Could you check a few things on this model? Use its own coordinates, in mm. A direction names the side the tool comes from. Give positions to 0.01 mm unless a question says otherwise; leave off trailing zeros. Loops run counter-clockwise (first coordinate to the right, second up) from the corner with the lowest first, then second, coordinate; pieces in that order, holes last.
1. For faces 4 (the conical face through (-17.686, 1.125, -29.712)), 5 (the cylindrical face through (19.122, 1.479, 33.174)), which set-ups out of +Z, -Z, +X, -X, +Y, -Y let a thin tool reach every point of the face, with its end or its side?
2. Imagine slicing it at D-D (z = -18). List the corners of the cut face in (x, y) for me.
3. I need wall thicknesses on line 1 along X through (y, z) = (1.45, -24.5); line 2 along X through (y, z) = (1.05, -18); line 3 along Z through (x, y) = (-15, 1.05). Which ranges of each line are inside material? Lowest first, please.
4. For P1, Ø2.5, axis at x = -32.5, z = 0, coming from the -Y side; P2, Ø6.5, axis at x = -16.25, z = 28.15, coming from the +Y side; P3, Ø4, axis at x = 42.44, z = 24.5, coming from the -Y side, each with a flat end and sliding along its axis, tell me the tip position at first contact or that it passes through.
5. Imagine slicing it at A-A (z = 0). List the corners of the cut face in (x, y) for me.
6. Thinking about a two-plate mould opening in X: for faces 1 (the flat face through (14, 1.52, -39.17)), 2 (the flat face through (3.12, 1.52, -36.86)), 3 (the flat face through (-22, 3, 22)), which applies, +X half, -X half, draft (parallel to the pull), parting line (faces both ways), or undercut?
7. Imagine slicing it at C-C (z = 49). List the corners of the cut face in (x, y) for me (3 decimals).
8. Imagine slicing it at B-B (x = -16.25). List the corners of the cut face in (y, z) for me.
```python
from build123d import *

# Parameters (mm, degrees)
SKETCH_1_R               = 52
SKETCH_1_R_2             = 1.525
SKETCH_1_R_3             = 2
SKETCH_1_R_4             = 27.5
EXTRUDE_1_DEPTH          = 3
HOLE_WIZARD_1_AT_2_COUNT = 2
HOLE_WIZARD_1_AT_2_PITCH = 32.5
HOLE_WIZARD_1_AT_3_COUNT = 2
HOLE_WIZARD_1_AT_3_PITCH = 56.291651246
HOLE_WIZARD_1_AT_4_COUNT = 2
HOLE_WIZARD_1_AT_4_PITCH = 65
HOLE_WIZARD_1_AT_5_COUNT = 2
HOLE_WIZARD_1_AT_5_PITCH = 56.291651246
HOLE_WIZARD_1_AT_6_COUNT = 2
HOLE_WIZARD_1_AT_6_PITCH = 32.5
CUT_EXTRUDE_1_DEPTH      = 10
FILLET_1_R               = 5
FILLET_2_R               = 1


with BuildPart() as part:
    # 草图1 → 凸台-拉伸1 (new body)
    with BuildSketch(Plane(origin=(0, 0, 0), x_dir=(1, 0, 0), z_dir=(0, 1, 0))):
        with Locations(Location((0, 0, 0), (0, 0, 270))):
            Circle(SKETCH_1_R)
        with Locations(Location((0, 49, 0), (0, 0, 270))):
            Circle(SKETCH_1_R_2, mode=Mode.SUBTRACT)
        with Locations(Location((-16.25, 28.145825623, 0), (0, 0, 270))):
            Circle(SKETCH_1_R_3, mode=Mode.SUBTRACT)
        with Locations(Location((42.435244785, 24.5, 0), (0, 0, 270))):
            Circle(SKETCH_1_R_2, mode=Mode.SUBTRACT)
        with Locations(Location((16.25, 28.145825623, 0), (0, 0, 270))):
            Circle(SKETCH_1_R_3, mode=Mode.SUBTRACT)
        with Locations(Location((42.435244785, -24.5, 0), (0, 0, 270))):
            Circle(SKETCH_1_R_2, mode=Mode.SUBTRACT)
        with Locations(Location((32.5, 0, 0), (0, 0, 270))):
            Circle(SKETCH_1_R_3, mode=Mode.SUBTRACT)
        with Locations(Location((0, -49, 0), (0, 0, 270))):
            Circle(SKETCH_1_R_2, mode=Mode.SUBTRACT)
        with Locations(Location((16.25, -28.145825623, 0), (0, 0, 270))):
            Circle(SKETCH_1_R_3, mode=Mode.SUBTRACT)
        with Locations(Location((-42.435244785, -24.5, 0), (0, 0, 270))):
            Circle(SKETCH_1_R_2, mode=Mode.SUBTRACT)
        with Locations(Location((-16.25, -28.145825623, 0), (0, 0, 270))):
            Circle(SKETCH_1_R_3, mode=Mode.SUBTRACT)
        with Locations(Location((-42.435244785, 24.5, 0), (0, 0, 270))):
            Circle(SKETCH_1_R_2, mode=Mode.SUBTRACT)
        with Locations(Location((-32.5, 0, 0), (0, 0, 270))):
            Circle(SKETCH_1_R_3, mode=Mode.SUBTRACT)
        with Locations(Location((0, 0, 0), (0, 0, 270))):
            Circle(SKETCH_1_R_4, mode=Mode.SUBTRACT)
    extrude(amount=EXTRUDE_1_DEPTH)

    # 草图3 → 孔1 (revolve, cut)
    with BuildSketch(Plane(origin=(-16.25, 3, -28.145825623), x_dir=(0, 0, 1), z_dir=(1, 0, 0))):
        Polygon((0, 0), (0, 3), (2, 3), (2, 2), (4, 0), align=None)
    hole_wizard_1 = revolve(axis=Axis((-16.25, 9.445314094, -28.145825623), (0, -1, 0)), mode=Mode.SUBTRACT)

    # 孔1 at 2: 孔1 ×2
    with Locations(*[(i * HOLE_WIZARD_1_AT_2_PITCH, 0, 0) for i in range(1, HOLE_WIZARD_1_AT_2_COUNT)]):
        add(hole_wizard_1, mode=Mode.SUBTRACT)

    # 孔1 at 3: 孔1 ×2
    with Locations(*[Vector(0.8660254037844387, 0, 0.5) * (i * HOLE_WIZARD_1_AT_3_PITCH) for i in range(1, HOLE_WIZARD_1_AT_3_COUNT)]):
        add(hole_wizard_1, mode=Mode.SUBTRACT)

    # 孔1 at 4: 孔1 ×2
    with Locations(*[Vector(0.5000000000000001, 0, 0.8660254037844386) * (i * HOLE_WIZARD_1_AT_4_PITCH) for i in range(1, HOLE_WIZARD_1_AT_4_COUNT)]):
        add(hole_wizard_1, mode=Mode.SUBTRACT)

    # 孔1 at 5: 孔1 ×2
    with Locations(*[(0, 0, i * HOLE_WIZARD_1_AT_5_PITCH) for i in range(1, HOLE_WIZARD_1_AT_5_COUNT)]):
        add(hole_wizard_1, mode=Mode.SUBTRACT)

    # 孔1 at 6: 孔1 ×2
    with Locations(*[Vector(-0.5000000000000003, 0, 0.8660254037844386) * (i * HOLE_WIZARD_1_AT_6_PITCH) for i in range(1, HOLE_WIZARD_1_AT_6_COUNT)]):
        add(hole_wizard_1, mode=Mode.SUBTRACT)

    # 草图5 → 切除-拉伸1 (cut)
    with BuildSketch(Plane(origin=(0, 3, 0), x_dir=(1, 0, 0), z_dir=(0, 1, 0))):
        with BuildLine():
            Line((-8.501262172, 46.22476113), (-18.947738206, 32.818445262))
            Line((-18.947738206, 32.818445262), (-35.781186336, 30.47468957))
            ThreePointArc((-35.781186336, 30.47468957), (-23.5, 40.703193978), (-8.501262172, 46.22476113))
        make_face()
        with BuildLine():
            Line((0, 40.865281716), (7.136483547, 31.706791111))
            ThreePointArc((7.136483547, 31.706791111), (0, 32.5), (-7.136483547, 31.706791111))
            Line((-7.136483547, 31.706791111), (0, 40.865281716))
        make_face()
        with BuildLine():
            Line((18.947738206, 32.818445262), (8.501262172, 46.22476113))
            ThreePointArc((8.501262172, 46.22476113), (23.5, 40.703193978), (35.781186336, 30.47468957))
            Line((35.781186336, 30.47468957), (18.947738206, 32.818445262))
        make_face()
        with BuildLine():
            Line((35.390372099, 20.432640858), (23.890644801, 22.033771601))
            ThreePointArc((23.890644801, 22.033771601), (28.145825623, 16.25), (31.027128348, 9.67301951))
            Line((31.027128348, 9.67301951), (35.390372099, 20.432640858))
        make_face()
        with BuildLine():
            Line((37.895476413, 0), (44.282448508, 15.75007156))
            ThreePointArc((44.282448508, 15.75007156), (47, 0), (44.282448508, -15.75007156))
            Line((44.282448508, -15.75007156), (37.895476413, 0))
        make_face()
        with BuildLine():
            Line((35.390372099, -20.432640858), (31.027128348, -9.67301951))
            ThreePointArc((31.027128348, -9.67301951), (28.145825623, -16.25), (23.890644801, -22.033771601))
            Line((23.890644801, -22.033771601), (35.390372099, -20.432640858))
        make_face()
        with BuildLine():
            Line((18.947738206, -32.818445262), (35.781186336, -30.47468957))
            ThreePointArc((35.781186336, -30.47468957), (23.5, -40.703193978), (8.501262172, -46.22476113))
            Line((8.501262172, -46.22476113), (18.947738206, -32.818445262))
        make_face()
        with BuildLine():
            Line((0, -40.865281716), (7.136483547, -31.706791111))
            ThreePointArc((7.136483547, -31.706791111), (0, -32.5), (-7.136483547, -31.706791111))
            Line((-7.136483547, -31.706791111), (0, -40.865281716))
        make_face()
        with BuildLine():
            Line((-18.947738206, -32.818445262), (-8.501262172, -46.22476113))
            ThreePointArc((-8.501262172, -46.22476113), (-23.5, -40.703193978), (-35.781186336, -30.47468957))
            Line((-35.781186336, -30.47468957), (-18.947738206, -32.818445262))
        make_face()
        with BuildLine():
            Line((-35.390372099, -20.432640858), (-23.890644801, -22.033771601))
            ThreePointArc((-23.890644801, -22.033771601), (-28.145825623, -16.25), (-31.027128348, -9.67301951))
            Line((-31.027128348, -9.67301951), (-35.390372099, -20.432640858))
        make_face()
        with BuildLine():
            Line((-37.895476413, 0), (-44.282448508, -15.75007156))
            ThreePointArc((-44.282448508, -15.75007156), (-47, 0), (-44.282448508, 15.75007156))
            Line((-44.282448508, 15.75007156), (-37.895476413, 0))
        make_face()
        with BuildLine():
            Line((-35.390372099, 20.432640858), (-31.027128348, 9.67301951))
            ThreePointArc((-31.027128348, 9.67301951), (-28.145825623, 16.25), (-23.890644801, 22.033771601))
            Line((-23.890644801, 22.033771601), (-35.390372099, 20.432640858))
        make_face()
    extrude(amount=-CUT_EXTRUDE_1_DEPTH, mode=Mode.SUBTRACT)

    # 圆角1
    fillet_1_edges = [part.edges().sort_by_distance(p)[0] for p in [
        (-18.947738206, 1.5, 32.818445262),
        (18.947738206, 1.5, 32.818445262),
        (37.895476413, 1.5, 0),
        (18.947738206, 1.5, -32.818445262),
        (-37.895476413, 1.5, 0),
        (-18.947738206, 1.5, -32.818445262),
    ]]
    fillet(fillet_1_edges, radius=FILLET_1_R)

    # 圆角2
    fillet_2_edges = [part.edges().sort_by_distance(p)[0] for p in [
        (-8.501262172, 1.5, 46.22476113),
        (-35.781186336, 1.5, 30.47468957),
        (0, 1.5, 40.865281716),
        (-7.136483547, 1.5, 31.706791111),
        (7.136483547, 1.5, 31.706791111),
        (35.781186336, 1.5, 30.47468957),
        (8.501262172, 1.5, 46.22476113),
        (35.390372099, 1.5, 20.432640858),
        (23.890644801, 1.5, 22.033771601),
        (31.027128348, 1.5, 9.67301951),
        (44.282448508, 1.5, -15.75007156),
        (44.282448508, 1.5, 15.75007156),
        (35.390372099, 1.5, -20.432640858),
        (31.027128348, 1.5, -9.67301951),
        (23.890644801, 1.5, -22.033771601),
        (8.501262172, 1.5, -46.22476113),
        (35.781186336, 1.5, -30.47468957),
        (-7.136483547, 1.5, -31.706791111),
        (0, 1.5, -40.865281716),
        (7.136483547, 1.5, -31.706791111),
        (-35.390372099, 1.5, -20.432640858),
        (-23.890644801, 1.5, -22.033771601),
        (-31.027128348, 1.5, -9.67301951),
        (-44.282448508, 1.5, 15.75007156),
        (-44.282448508, 1.5, -15.75007156),
        (-35.390372099, 1.5, 20.432640858),
        (-31.027128348, 1.5, 9.67301951),
        (-23.890644801, 1.5, 22.033771601),
        (-35.781186336, 1.5, -30.47468957),
        (-8.501262172, 1.5, -46.22476113),
    ]]
    fillet(fillet_2_edges, radius=FILLET_2_R)


solid = part.part
```
Derived:
1. face 4: +Y
1. face 5: +Y, -Y
2. outline: (-48.79, 0) - (-34.4, 0) - (-34.4, 3) - (-48.79, 3) - close; (-27.06, 0) - (-20.79, 0) - (-20.79, 3) - (-27.06, 3) - close; (20.79, 0) - (27.06, 0) - (27.06, 3) - (20.79, 3) - close; (34.4, 0) - (48.79, 0) - (48.79, 3) - (34.4, 3) - close
3. line 1: x = -45.87 to -43.96, -40.91 to -12.49, 12.49 to 40.91, 43.96 to 45.87
3. line 2: x = -48.79 to -34.4, -27.06 to -20.79, 20.79 to 27.06, 34.4 to 48.79
3. line 3: z = -49.79 to -44.54, -37.88 to -29.77, -26.52 to -23.05, 23.05 to 26.52, 29.77 to 37.88, 44.54 to 49.79
4. P1: passes through
4. P2: stops at y = 2.25
4. P3: stops at y = 0
5. outline: (-52, 0) - (-47, 0) - (-47, 3) - (-52, 3) - close; (-38.29, 0) - (-34.5, 0) - (-34.5, 1) - (-36.5, 3) - (-38.29, 3) - close; (-30.5, 0) - (-27.5, 0) - (-27.5, 3) - (-28.5, 3) - (-30.5, 1) - close; (27.5, 0) - (30.5, 0) - (30.5, 1) - (28.5, 3) - (27.5, 3) - close; (34.5, 0) - (38.29, 0) - (38.29, 3) - (36.5, 3) - (34.5, 1) - close; (47, 0) - (52, 0) - (52, 3) - (47, 3) - close
6. face 1: undercut
6. face 2: undercut
6. face 3: draft
7. outline: (-17.407, 0) - (-1.525, 0) - (-1.525, 3) - (-17.407, 3) - close; (1.525, 0) - (17.407, 0) - (17.407, 3) - (1.525, 3) - close
8. outline: (0, -49.4) - (3, -49.4) - (3, -44.1) - (0, -44.1) - close; (0, -36.28) - (3, -36.28) - (3, -32.15) - (1, -30.15) - (0, -30.15) - close; (0, -26.15) - (1, -26.15) - (3, -24.15) - (3, -22.19) - (0, -22.19) - close; (0, 22.19) - (3, 22.19) - (3, 24.15) - (1, 26.15) - (0, 26.15) - close; (0, 30.15) - (1, 30.15) - (3, 32.15) - (3, 36.28) - (0, 36.28) - close; (0, 44.1) - (3, 44.1) - (3, 49.4) - (0, 49.4) - close
